Could you check a few things on this model? Use its own coordinates, in mm. A direction names the side the tool comes from. Round coordinates to 2 decimals unless told otherwise and drop trailing zeros. Loops run counter-clockwise (first coordinate to the right, second up) from the corner with the lowest first, then second, coordinate; pieces in that order, holes last.
from build123d import *

# Parameters (mm, degrees)
BOSS_EXTRUDE1_DEPTH = 31.75
SKETCH3_R           = 3.3782
CUT_EXTRUDE1_DEPTH  = 7.35


with BuildPart() as part:
    # Sketch1 → Boss-Extrude1 (new body)
    with BuildSketch(Plane.XY):
        with BuildLine():
            Line((12.475198354, 6.35), (0, 6.35))
            Line((0, 6.35), (0, 0))
            Line((0, 0), (17.78, 0))
            ThreePointArc((17.78, 0), (31.242, 13.462), (44.704, 0))
            Line((44.704, 0), (76.2, 0))
            ThreePointArc((76.2, 0), (89.662, 13.462), (103.124, 0))
            Line((103.124, 0), (120.904, 0))
            Line((120.904, 0), (120.904, 6.35))
            Line((120.904, 6.35), (108.428801646, 6.35))
            ThreePointArc((108.428801646, 6.35), (89.662, 19.812), (70.895198354, 6.35))
            Line((70.895198354, 6.35), (50.008801646, 6.35))
            ThreePointArc((50.008801646, 6.35), (31.242, 19.812), (12.475198354, 6.35))
        make_face()
    extrude(amount=BOSS_EXTRUDE1_DEPTH)

    # Sketch3 → Cut-Extrude1 (cut, through all)
    with BuildSketch(Plane(origin=(0, 6.35, 0), x_dir=(1, 0, 0), z_dir=(0, 1, 0))):
        with Locations((6.237599177, -15.875)):
            Circle(SKETCH3_R)
        with Locations((60.452, -15.875)):
            Circle(SKETCH3_R)
        with Locations((114.666400823, -15.875)):
            Circle(SKETCH3_R)
    extrude(amount=-CUT_EXTRUDE1_DEPTH, mode=Mode.SUBTRACT)


solid = part.part
Item 1: If we section it at C-C, the plane z = 18: Please give me the cut outline in (x, y), then the cut area to 3 significant figures.
Results list:
outline: (0, 0) - (3.61, 0) - (3.61, 6.35) - (0, 6.35) - close; (8.86, 0) - (17.78, 0) arc R13.46 cw to (44.7, 0) - (57.83, 0) - (57.83, 6.35) - (50.01, 6.35) arc R19.81 ccw to (12.48, 6.35) - (8.86, 6.35) - close; (63.08, 0) - (76.2, 0) arc R13.46 cw to (103.12, 0) - (112.04, 0) - (112.04, 6.35) - (108.43, 6.35) arc R19.81 ccw to (70.9, 6.35) - (63.08, 6.35) - close; (117.29, 0) - (120.9, 0) - (120.9, 6.35) - (117.29, 6.35) - close
area: 837 mm2
Item 2: If we section it at B-B, the plane z = 28: Please give me the cut outline in (x, y), then the cut area to 3 significant figures.
Results list:
outline: (0, 0) - (17.78, 0) arc R13.46 cw to (44.7, 0) - (76.2, 0) arc R13.46 cw to (103.12, 0) - (120.9, 0) - (120.9, 6.35) - (108.43, 6.35) arc R19.81 ccw to (70.9, 6.35) - (50.01, 6.35) arc R19.81 ccw to (12.48, 6.35) - (0, 6.35) - close
area: 937 mm2
Item 3: If we section it at A-A, the plane y = 8.75: Please give me the cut outline in (x, z), then the cut area to 3 significant figures.
Results list:
outline: (13.47, 0) - (21.01, 0) - (21.01, 31.75) - (13.47, 31.75) - close; (41.47, 0) - (49.02, 0) - (49.02, 31.75) - (41.47, 31.75) - close; (71.89, 0) - (79.43, 0) - (79.43, 31.75) - (71.89, 31.75) - close; (99.89, 0) - (107.44, 0) - (107.44, 31.75) - (99.89, 31.75) - close
area: 958 mm2
Item 4: For faces 5 (the flat face through (6, 6.35, 12)), 6 (the flat face through (0, 3, 16)), 7 (the flat face through (115, 6.35, 12)), which set-ups out of +Z, -Z, +X, -X, +Y, -Y let a thin tool reach every point of the face, with its end or its side?
Results list:
face 5: +Z, -Z, -X, +Y
face 6: +Z, -Z, -X, +Y, -Y
face 7: +Z, -Z, +X, +Y
Item 5: If I drill on line 1 along X through (y, z) = (2, 16.5); line 2 along X through (y, z) = (9.5, 27); line 3 along X through (y, z) = (6.75, 1), over which ranges is the centre line in solid material (lowest first)?
Results list:
line 1: x = 0 to 2.92, 9.56 to 17.93, 44.55 to 57.13, 63.77 to 76.35, 102.97 to 111.35, 117.99 to 120.9
line 2: x = 13.86 to 21.7, 40.78 to 48.63, 72.28 to 80.12, 99.2 to 107.05
line 3: x = 12.62 to 19.59, 42.89 to 49.87, 71.04 to 78.01, 101.31 to 108.29
Item 6: We'd pull the mould along Z, two halves only. Please class faces 1 (the flat face through (60, 6, 0)), 2 (the flat face through (61, 6.35, 12)), 3 (the cylindrical face through (62.27, 3.22, 13.03)), 4 (the flat face through (60, 6, 31.75)): released by +Z, released by -Z, zero draft, split by the parting line, or undercut.
Results list:
face 1: released by -Z
face 2: zero draft
face 3: undercut
face 4: released by +Z
Item 7: If we section it at D-D, the plane x = 55: Please give me the cut outline in (y, z).
Results list:
outline: (0, 0) - (6.35, 0) - (6.35, 31.75) - (0, 31.75) - close
Item 8: Will these pins go through, and if not, where does the flat tip stop? pin 1 (10 mm diameter, centred on x = 115, z = 22.5, fed in from +Y); pin 2 (6 mm diameter, centred on x = 28.5, z = 12, fed in from +Y); pin 3 (10 mm diameter, centred on x = 17.5, z = 7, fed in from +Y).
Results list:
pin 1: stops at y = 6.35
pin 2: stops at y = 19.81
pin 3: stops at y = 17.78
